```python
from build123d import *

# Parameters (mm, degrees)
SKETCH4_W                = 12.46
SKETCH4_H                = 17.25
BOSS_EXTRUDE3_DEPTH      = 6
SKETCH8_R                = 12.546781182
SKETCH8_R_2              = 11.15
BOSS_EXTRUDE6_DEPTH      = 7.3
BOSS_EXTRUDE6_DEPTH_BACK = 17.25
BOSS_EXTRUDE4_DEPTH      = 17.25
SKETCH6_R                = 0.5
CUT_EXTRUDE1_DEPTH       = 15
CHAMFER1_SIZE            = 0.5
CHAMFER1_SIZE2           = 0.866025404
SKETCH10_W               = 12.46
SKETCH10_H               = 23.7
CUT_EXTRUDE3_DEPTH       = 17.25
CUT_EXTRUDE4_REACH       = 38.097
SKETCH11_W               = 5
SKETCH11_H               = 3
BOSS_EXTRUDE7_DEPTH      = 7.3
BOSS_EXTRUDE9_DEPTH      = 10
SKETCH20_R               = 11.15
SKETCH20_R_2             = 7.15
BOSS_EXTRUDE11_DEPTH     = 7.3
SKETCH21_R               = 10.15
SKETCH21_R_2             = 7.15
CUT_EXTRUDE7_DEPTH       = 1.3
BOSS_EXTRUDE10_DEPTH     = 34.55
SKETCH18_W               = 20
SKETCH18_H               = 12.438292938
CUT_EXTRUDE5_DEPTH       = 2
SKETCH19_R               = 1.25
CUT_EXTRUDE6_DEPTH       = 53.296781182
CUT_EXTRUDE6_DEPTH_BACK  = 3
FILLET1_R                = 10
SKETCH22_R               = 5.8
BOSS_EXTRUDE12_DEPTH     = 20
FILLET2_R                = 2
SKETCH23_R               = 5.930854157
SKETCH23_R_2             = 5.08
CUT_EXTRUDE8_DEPTH       = 11.6
SKETCH24_R               = 6.5
BOSS_EXTRUDE13_DEPTH     = 2
SKETCH25_R               = 1.25
BOSS_EXTRUDE14_DEPTH     = 2
SKETCH26_W               = 5
SKETCH26_H               = 3
BOSS_EXTRUDE15_DEPTH     = 5


with BuildPart() as part:
    # Sketch4 → Boss-Extrude3 (new body)
    with BuildSketch(Plane.XY):
        with Locations((0, -1.35)):
            Rectangle(SKETCH4_W, SKETCH4_H)
    extrude(amount=BOSS_EXTRUDE3_DEPTH)



with BuildPart() as body_2:
    # Sketch8 → Boss-Extrude6 (new body, two sides)
    with BuildSketch(Plane(origin=(0, -9.975, 0), x_dir=(-1, 0, 0), z_dir=(0, -1, 0))) as boss_extrude6_sk:
        with Locations((0, -23.55)):
            Circle(SKETCH8_R)
        with Locations((0, -23.55)):
            Circle(SKETCH8_R_2, mode=Mode.SUBTRACT)
    extrude(amount=BOSS_EXTRUDE6_DEPTH)
    extrude(boss_extrude6_sk.sketch, amount=-BOSS_EXTRUDE6_DEPTH_BACK)


with BuildPart() as part_1:
    add(part.part)

    add(body_2.part)  # Boss-Extrude4 merges body 2
    # Sketch5 → Boss-Extrude4 (add)
    with BuildSketch(Plane(origin=(0, 7.275, 0), x_dir=(1, 0, 0), z_dir=(0, 1, 0))):
        with BuildLine():
            Line((12.546781182, -23.55), (12.546781182, 0))
            Line((12.546781182, 0), (6.23, 0))
            Line((6.23, 0), (6.23, -29.7))
            Line((6.23, -29.7), (-6.23, -29.7))
            Line((-6.23, -29.7), (-6.23, 0))
            Line((-6.23, 0), (-12.546781182, 0))
            Line((-12.546781182, 0), (-12.546781182, -23.55))
            ThreePointArc((-12.546781182, -23.55), (0, -36.096781182), (12.546781182, -23.55))
        make_face()
    extrude(amount=-BOSS_EXTRUDE4_DEPTH)

    # Sketch6 → Cut-Extrude1 (cut)
    with BuildSketch(Plane(origin=(0, 7.275, 0), x_dir=(1, 0, 0), z_dir=(0, 1, 0))):
        with Locations((0, -3.6)):
            Circle(SKETCH6_R)
        with Locations((0, -32.1)):
            Circle(SKETCH6_R)
    extrude(amount=-CUT_EXTRUDE1_DEPTH, mode=Mode.SUBTRACT)

    # Chamfer1
    chamfer1_edges = [part_1.edges().sort_by_distance(p)[0] for p in [
        (-0.5, 7.275, 3.6),
        (-0.5, 7.275, 32.1),
    ]]
    chamfer1_side = [part_1.faces().sort_by_distance(p)[0] for p in [
        (0, 7.275, 35.657160381),
    ]]
    chamfer(chamfer1_edges, length=CHAMFER1_SIZE, length2=CHAMFER1_SIZE2, reference=chamfer1_side[0])

    # Sketch10 → Cut-Extrude3 (cut)
    with BuildSketch(Plane(origin=(0, 7.275, 0), x_dir=(1, 0, 0), z_dir=(0, 1, 0))):
        with Locations((0, -17.85)):
            Rectangle(SKETCH10_W, SKETCH10_H)
    extrude(amount=-CUT_EXTRUDE3_DEPTH, mode=Mode.SUBTRACT)

    # Sketch11 → Cut-Extrude4 (cut, up to next)
    with BuildSketch(Plane.XY.offset(36.096781182), mode=Mode.PRIVATE) as cut_extrude4_sk1:
        with Locations((0, -8.475)):
            Rectangle(SKETCH11_W, SKETCH11_H)
    cut_extrude4_tool1 = extrude(cut_extrude4_sk1.sketch, amount=-CUT_EXTRUDE4_REACH, mode=Mode.PRIVATE) & part_1.part
    add(cut_extrude4_tool1.solids().sort_by_distance((0, -8.475, 36.096781))[0], mode=Mode.SUBTRACT)

    # Sketch13 → Boss-Extrude7 (add)
    with BuildSketch(Plane.XZ.offset(17.275)):
        with BuildLine():
            Line((-12.546781182, 23.55), (-12.546781182, 0))
            Line((-12.546781182, 0), (12.546781182, 0))
            Line((12.546781182, 0), (12.546781182, 23.55))
            ThreePointArc((12.546781182, 23.55), (0, 11.003218818), (-12.546781182, 23.55))
        make_face()
    extrude(amount=-BOSS_EXTRUDE7_DEPTH)

    # Sketch15 → Boss-Extrude9 (add)
    with BuildSketch(Plane(origin=(0, 7.275, 0), x_dir=(1, 0, 0), z_dir=(0, 1, 0))):
        with BuildLine():
            Line((-12.546781182, 0), (12.546781182, 0))
            Line((12.546781182, 0), (12.546781182, -23.55))
            ThreePointArc((12.546781182, -23.55), (0, -36.096781182), (-12.546781182, -23.55))
            Line((-12.546781182, -23.55), (-12.546781182, 0))
        make_face()
        with BuildLine():
            Line((-6.23, -0.8), (6.23, -0.8))
            Line((6.23, -0.8), (6.23, -33.5))
            ThreePointArc((6.23, -33.5), (5.937106781, -34.207106781), (5.23, -34.5))
            Line((5.23, -34.5), (-5.23, -34.5))
            ThreePointArc((-5.23, -34.5), (-5.937106781, -34.207106781), (-6.23, -33.5))
            Line((-6.23, -33.5), (-6.23, -0.8))
        make_face(mode=Mode.SUBTRACT)
    extrude(amount=BOSS_EXTRUDE9_DEPTH)

    # Sketch20 → Boss-Extrude11 (add)
    with BuildSketch(Plane.XZ.offset(17.275)):
        with Locations((0, 23.55)):
            Circle(SKETCH20_R)
        with Locations((0, 23.55)):
            Circle(SKETCH20_R_2, mode=Mode.SUBTRACT)
    extrude(amount=-BOSS_EXTRUDE11_DEPTH)

    # Sketch21 → Cut-Extrude7 (cut)
    with BuildSketch(Plane.XZ.offset(17.275)):
        with Locations((0, 23.55)):
            Circle(SKETCH21_R)
        with Locations((0, 23.55)):
            Circle(SKETCH21_R_2, mode=Mode.SUBTRACT)
    extrude(amount=-CUT_EXTRUDE7_DEPTH, mode=Mode.SUBTRACT)

    # Sketch17 → Boss-Extrude10 (add)
    with BuildSketch(Plane(origin=(0, 17.275, 0), x_dir=(1, 0, 0), z_dir=(0, 1, 0))):
        Polygon((21.75, 25), (21.75, 0), (-32.546781182, 0), (-32.546781182, 25), (-28.546781182, 25), (-28.546781182, 5), (17.75, 5), (17.75, 25), align=None)
    extrude(amount=-BOSS_EXTRUDE10_DEPTH)

    # Sketch18 → Cut-Extrude5 (cut)
    with BuildSketch(Plane.ZY.offset(-17.75)):
        with Locations((-15, 0)):
            Rectangle(SKETCH18_W, SKETCH18_H)
    extrude(amount=-CUT_EXTRUDE5_DEPTH, mode=Mode.SUBTRACT)

    # Sketch19 → Cut-Extrude6 (cut, two sides)
    with BuildSketch(Plane.ZY.offset(-19.75)) as cut_extrude6_sk:
        with Locations((-20, 0)):
            Circle(SKETCH19_R)
    extrude(amount=CUT_EXTRUDE6_DEPTH, mode=Mode.SUBTRACT)
    extrude(cut_extrude6_sk.sketch, amount=-CUT_EXTRUDE6_DEPTH_BACK, mode=Mode.SUBTRACT)

    # Fillet1
    fillet1_edges = [part_1.edges().sort_by_distance(p)[0] for p in [
        (19.75, 17.275, -25),
        (-30.546781182, 17.275, -25),
        (-30.546781182, -17.275, -25),
        (19.75, -17.275, -25),
    ]]
    fillet(fillet1_edges, radius=FILLET1_R)

    # Sketch22 → Boss-Extrude12 (add)
    with BuildSketch(Plane(origin=(-28.546781182, 0, 0), x_dir=(0, 0, -1), z_dir=(1, 0, 0))):
        with Locations((20, 0)):
            Circle(SKETCH22_R)
    extrude(amount=BOSS_EXTRUDE12_DEPTH)

    # Fillet2
    fillet2_edges = [part_1.edges().sort_by_distance(p)[0] for p in [
        (-8.546781182, 0, -14.2),
    ]]
    fillet(fillet2_edges, radius=FILLET2_R)

    # Sketch23 → Cut-Extrude8 (cut)
    with BuildSketch(Plane(origin=(-28.546781182, 0, 0), x_dir=(0, 0, -1), z_dir=(1, 0, 0))):
        with Locations((20, 0)):
            Circle(SKETCH23_R)
        with Locations((20, 0)):
            Circle(SKETCH23_R_2, mode=Mode.SUBTRACT)
    extrude(amount=CUT_EXTRUDE8_DEPTH, mode=Mode.SUBTRACT)

    # Sketch24 → Boss-Extrude13 (add)
    with BuildSketch(Plane.ZY.offset(16.946781182)):
        with Locations((-20, 0)):
            Circle(SKETCH24_R)
    extrude(amount=BOSS_EXTRUDE13_DEPTH)

    # Sketch25 → Boss-Extrude14 (add)
    with BuildSketch(Plane.ZY.offset(32.546781182)):
        with Locations((-20, 0)):
            Circle(SKETCH25_R)
    extrude(amount=-BOSS_EXTRUDE14_DEPTH)

    # Sketch26 → Boss-Extrude15 (add)
    with BuildSketch(Plane(origin=(-28.546781182, 0, 0), x_dir=(0, 0, -1), z_dir=(1, 0, 0))):
        with Locations((7.5, -8.275)):
            Rectangle(SKETCH26_W, SKETCH26_H)
        with Locations((7.5, -3.759)):
            Rectangle(SKETCH26_W, SKETCH26_H)
    extrude(amount=BOSS_EXTRUDE15_DEPTH)


solid = part_1.part
```
CAD build for the part. Positions are in the model's coordinates, mm. A direction names the side the tool comes from. Round coordinates to 2 decimals unless told otherwise and drop trailing zeros. Loops run counter-clockwise (first coordinate to the right, second up) from the corner with the lowest first, then second, coordinate; pieces in that order, holes last. Notation, with made-up numbers: (81, 26.25) - (117, 26.25) arc R26 ccw to (117, 51.25) - close; hole circle Ø4 at (53, -39.5). An arc over 180 degrees is marked (long way). Return JSON: item names as keys, results as strings. Group by question number.
Q1. Flat gauge pins, fed straight in: pin 1 Ø2 at (y, z) = (8.5, 13) entering from +X; pin 2 Ø6 at (x, z) = (-19, -14.5) entering from -Y; pin 3 Ø13.5 at (x, y) = (-0.5, -1.5) entering from -Z. Where does each tip first touch, or does it go through?
Q2. Drill centre lines: line 1 along Z through (x, y) = (0, 0); line 2 along X through (y, z) = (3.25, 3.6); line 3 along Z through (x, y) = (-29.95, 0). Where is each one in solid material? Low to high. Write a range as [from, to].
Q3. Two-plate mould, pull along Y, no slides. Class faces 1 (the face through (-29.533, -0.479, -18.845)), 2 (the face through (17, 0, 0)), 3 (the face through (0, -9.975, 12)): +Y half, -Y half, draft (parallel to the pull), parting line (faces both ways), or undercut.
Q4. Band-saw the part on D-D on x = 18.5. Give the cut face in (y, z) (3 decimals), plus the area to 3 significant figures.
Q5. Tool access for faces 4 (the face through (-22, 0, 0)), 5 (the face through (-30.547, 0, -20)), 6 (the face through (2.5, -8, 33)), 7 (the face through (19, -6.219, -15)): list every direction of +Z, -Z, +X, -X, +Y, -Y with a clear straight run to the whole face (end or side of a thin tool).
Q6. Band-saw the part on C-C on z = -12.5. Give the cut face in (x, y) (3 decimals).
Q7. Band-saw the part on A-A on z = -20. Give the number of separate pieces and of enclosed holes in the cut face, plus the area to 3 significant figures.
Q8. Band-saw the part on B-B on x = -15.5. Give the cut face in (y, z) (3 decimals).
Solutions:
{
 "1": {"pin 1": "stops at x = 12.55", "pin 2": "stops at y = -6", "pin 3": "stops at z = -5"},
 "2": {"line 1": "z = [-5, 3.1], [4.1, 6], [29.7, 31.6], [32.6, 36.1]", "line 2": "x = [-12.55, -0.5], [0.5, 12.55]", "line 3": "z = [-25, -21.25], [-18.75, 0]"},
 "3": {"face 1": "undercut", "face 2": "draft", "face 3": "+Y half"},
 "4": {"outline": "(-17.275, -15) arc R10 ccw to (-7.275, -25) - (-6.219, -25) - (-6.219, -5) - (6.219, -5) - (6.219, -25) - (7.275, -25) arc R10 ccw to (17.275, -15) - (17.275, 0) - (-17.275, 0) - close", "area": "572 mm^2"},
 "5": {"face 4": "+Z, -X, +Y, -Y", "face 5": "none", "face 6": "+Z", "face 7": "-Z"},
 "6": {"outline": "(-32.547, -17.275) - (-28.547, -17.275) - (-28.547, 17.275) - (-32.547, 17.275) - close; (17.75, -17.275) - (21.75, -17.275) - (21.75, 17.275) - (17.75, 17.275) - (17.75, 6.219) - (19.75, 6.219) - (19.75, -6.219) - (17.75, -6.219) - close"},
 "7": {"separate pieces": "3", "enclosed holes": "1", "area": "439 mm^2"},
 "8": {"outline": "(-17.275, -5) - (17.275, -5) - (17.275, 0) - (-17.275, 0) - close; circle Ø11.6 at (0, -20)"}
}
